Design review of the part built by this model. Coordinates are the model's own, in mm. Coordinates: 2 decimals unless noted, no trailing zeros. Loops run counter-clockwise (first coordinate to the right, second up) from the corner with the lowest first, then second, coordinate; pieces in that order, holes last. Notation, with made-up numbers: (67, 14) - (75, 14) arc R24 cw to (75, 29) - close; hole circle Ø4 at (68, 39.25). An arc over 180 degrees is marked (long way). Answer in a Markdown table with one row per item. Add a question column.
(1) To check wall thickness, follow L1, parallel to Z at x = 0, y = -2.1; L2, parallel to X at y = -2.35, z = 1.25; L3, parallel to X at y = -1.95, z = 0.75. State the ranges of each line that lie inside material, in increasing order. Write a range as [from, to].
(2) We need section D-D, the plane x = 2.75. Write out the cut boundary in (y, z).
(3) We need section A-A, the plane x = 0. Write out the cut boundary in (y, z).
(4) We need section B-B, the plane y = -2.45. Write out the cut boundary in (x, z).
(5) The part is to be moulded in two halves that separate along Z. For faces 1 (the face through (2.003, -2.024, 0.631)), 2 (the face through (2, -4, 2)), 3 (the face through (3.26, -3.85, 1.85)), 4 (the face through (3.23, -0.15, -1.9)), say which applies: released by +Z, released by -Z, zero draft, split by the parting line, or undercut.
(6) We need section C-C, the plane z = 2.75. Write out the cut boundary in (x, y), plus the area to 3 significant figures.
from build123d import *

# Parameters (mm, degrees)
F1_DEPTH = 4
F3_D     = 4.2
F4_SIZE  = 0.3


with BuildPart() as f1:
    # F0 (on Front) → F1 (new body)
    with BuildSketch(Plane.XZ):
        Polygon((2.2516660498, 3.9), (-2.2516660498, 3.9), (-4.5033320997, 0), (-2.2516660498, -3.9), (2.2516660498, -3.9), (4.5033320997, 0), align=None)
    extrude(amount=F1_DEPTH)

    # F3 (through all)
    with Locations(Plane(origin=(0, 0, 0), x_dir=(-1, 0, 0), z_dir=(0, 1, 0))):
        with Locations((0, 0)):
            Hole(F3_D / 2)

    # F4
    f4_edges = [f1.edges().sort_by_distance(p)[0] for p in [
        (0, 0, -3.9),
        (-3.377499, 0, -1.95),
        (0, 0, 3.9),
        (-3.377499, 0, 1.95),
        (3.377499, 0, 1.95),
        (3.377499, 0, -1.95),
        (2.1, 0, 0),
        (3.377499, -4, 1.95),
        (3.377499, -4, -1.95),
        (0, -4, 3.9),
        (0, -4, -3.9),
        (-3.377499, -4, 1.95),
        (-3.377499, -4, -1.95),
        (2.1, -4, 0),
    ]]
    chamfer(f4_edges, length=F4_SIZE)


solid = f1.part
Responses:
| question | item | result |
|---|---|---|
| 1 | L1 | z = [-3.9, -2.1], [2.1, 3.9] |
| 1 | L2 | x = [-3.78, -1.69], [1.69, 3.78] |
| 1 | L3 | x = [-4.07, -1.96], [1.96, 4.07] |
| 2 | outline | (-4, -2.44) - (-3.7, -3.04) - (-0.3, -3.04) - (0, -2.44) - (0, 2.44) - (-0.3, 3.04) - (-3.7, 3.04) - (-4, 2.44) - close |
| 3 | outline | (-4, -3.6) - (-3.7, -3.9) - (-0.3, -3.9) - (0, -3.6) - (0, -2.4) - (-0.3, -2.1) - (-3.7, -2.1) - (-4, -2.4) - close; (-4, 2.4) - (-3.7, 2.1) - (-0.3, 2.1) - (0, 2.4) - (0, 3.6) - (-0.3, 3.9) - (-3.7, 3.9) - (-4, 3.6) - close |
| 4 | outline | (-4.5, 0) - (-2.25, -3.9) - (2.25, -3.9) - (4.5, 0) - (2.25, 3.9) - (-2.25, 3.9) - close; hole circle Ø4.2 at (0, 0) |
| 5 | face 1 | undercut |
| 5 | face 2 | zero draft |
| 5 | face 3 | released by +Z |
| 5 | face 4 | released by -Z |
| 6 | outline | (-2.92, -3.7) - (-2.57, -4) - (2.57, -4) - (2.92, -3.7) - (2.92, -0.3) - (2.57, 0) - (-2.57, 0) - (-2.92, -0.3) - close |
| 6 | area | 23.1 mm2 |
